Could you check a few things on this model? Use its own coordinates, in mm. A direction names the side the tool comes from. Coordinates: 2 decimals unless noted, no trailing zeros. Write each loop counter-clockwise with the first axis right and the second up, starting at its lowest first coordinate (ties: lowest second). Pieces come first, ordered by that corner, then holes. Notation, with made-up numbers: M 66,14.5 L 85,14.5 A12 cw 85,25.5 Z; hole C 78.5,54.25 d1. An arc over 180 degrees is marked long. Answer as CSV lines item,"result". Start each with the question number.
Item 1: Suppose I cut it at A-A, the plane z = 6.75. Write out the boundary of the cut face in (x, y).
Item 2: Suppose I cut it at C-C, the plane z = 12.5. Write out the boundary of the cut face in (x, y), and give its area (3 significant figures).
Item 3: We'd pull the mould along X, two halves only. Please class faces 1 (the cylindrical face through (3.52, -1.46, 3.76)), 2 (the flat face through (0, 0, 0)), 3 (the cylindrical face through (1.817, -0.053, 4.382)): +X half, -X half, draft (parallel to the pull), parting line (faces both ways), or undercut.
Item 4: On a 3-axis mill with a long thin cutter (end or side, diameter ignored), from which of +Z, -Z, +X, -X, +Y, -Y can I reach the whole of each face in a straight line? I mean faces 4 (the cylindrical face through (-1.05, -0.8, 14.41)), 5 (the flat face through (0, 0, 17.78)). Say none if no direction works.
Item 5: I'm going to push flat-ended pins straight in: P1, Ø2, axis at x = 2.5, y = 2, coming from the -Z side; P2, Ø2, axis at x = 0, z = 13.5, coming from the -Y side. Where does each tip first touch, or does it pass through?
Item 6: If I drill on line 1 along Z through (x, y) = (0, 0.5) (3 decimals); line 2 along X through (y, z) = (1.75, 3.81) (3 decimals); line 3 along X through (y, z) = (-1, 3.81) (3 decimals), over which ranges is the centre line in solid material (lowest first)? Write a range as [from, to].
Item 7: Suppose I cut it at B-B, the plane z = 3.81. Write out the boundary of the cut face in (x, y) (3 decimals).
```python
from build123d import *

# Parameters (mm, degrees)
F0_R          = 3.81
F0_R_2        = 1.3208
F1_DEPTH      = 7.62
F2_DEPTH      = 17.78
F3_R          = 1.905
F4_DEPTH      = 25.4
F4_DEPTH_BACK = 25.4


with BuildPart() as f1:
    # F0 (on Top) → F1 (new body)
    with BuildSketch(Plane.XY):
        Circle(F0_R)
        Circle(F0_R_2, mode=Mode.SUBTRACT)
        Circle(F0_R_2)
    extrude(amount=F1_DEPTH)

    # F0 (on Top) → F2 (join)
    with BuildSketch(Plane.XY):
        Circle(F0_R_2)
    extrude(amount=F2_DEPTH)

    # F3 (on Front) → F4 (cut, two sides)
    with BuildSketch(Plane.XZ) as f4_sk:
        with Locations((0, 3.81)):
            Circle(F3_R)
    extrude(amount=-F4_DEPTH, mode=Mode.SUBTRACT)
    extrude(f4_sk.sketch, amount=F4_DEPTH_BACK, mode=Mode.SUBTRACT)

    # F5 (on Front) → F6 (revolve)
    with BuildSketch(Plane.XZ):
        with BuildLine():
            Line((0, 15.0378467515), (0, 7.62))
            Line((0, 7.62), (3.81, 7.62))
            add(Edge.make_bspline(
                [(3.81, 7.62), (1.0146183195, 8.7640155107), (1.5803196002, 12.1609568596), (0, 15.0378467515)],
                knots=[0, 0, 0, 0, 8.3390976987, 8.3390976987, 8.3390976987, 8.3390976987], degree=3))
        make_face()
    revolve(axis=Axis((0, 0, 17.78), (0, 0, 1)))


solid = f1.part
```
Ans:
1,outline,"C 0,0 d7.62"
2,outline,"C 0,0 d2.64"
2,area,"5.48 mm^2"
3,face 1,"parting line"
3,face 2,"draft"
3,face 3,"undercut"
4,face 4,"+Z"
4,face 5,"+Z, +X, -X, +Y, -Y"
5,P1,"stops at z = 0"
5,P2,"stops at y = -1.32"
6,line 1,"z = [0, 1.905], [5.715, 17.78]"
6,line 2,"x = [-3.384, -1.905], [1.905, 3.384]"
6,line 3,"x = [-3.676, -1.905], [1.905, 3.676]"
7,outline,"M -1.905,-3.3 L -1.905,3.3 A3.81 ccw Z; M 1.905,-3.3 A3.81 ccw 1.905,3.3 Z"
